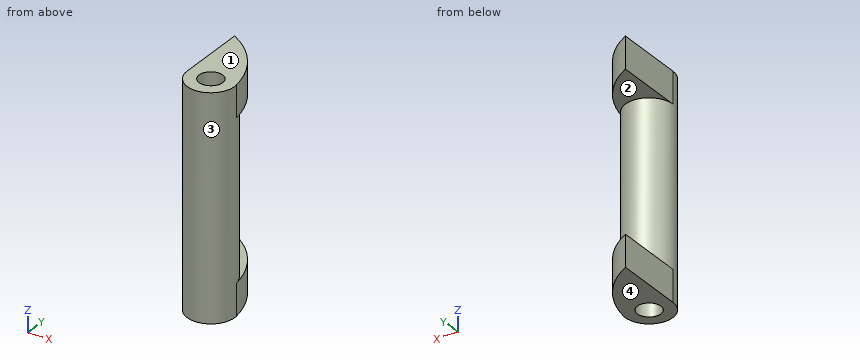
Autodesk Inventor part; units mm, degrees
ref_plane "YZ Plane" through (0, 0, 0) normal (1, 0, 0) x (0, 1, 0)
ref_plane "XZ Plane" through (0, 0, 0) normal (0, 1, 0) x (-1, 0, 0)
sketch "草图1" plane through (0, 0, 0) normal (0, 0, 1) x (1, 0, 0)
  circle A0 centre (0, 0) radius 1.5
  circle A1 centre (0, 0) radius 3
  line L0 (-3, 0) -> (-3, 9)
  arc A2 (2.9736, 0.3973) -> (-3, 9) centre (-8.3955, -1.1218) ccw
  dimension "d0" = 3
  dimension "d1" = 6
  dimension "d2" = 9
sketch "草图2" plane through (0, 0, 0) normal (0, 1, 0) x (-1, 0, 0)
  line L0 (3, 0) -> (3, -28)
  line L1 (3, 0) -> (3, -4)
  line L2 (3, -28) -> (3, -24)
  point P0 (0, 0)
  point P1 (3, -14)
  dimension "d3" = 28
  dimension "d6" = 4
  dimension "d7" = 4
extrude "拉伸1" add sketch "草图1" against normal blind 28 contours A1
extrude "拉伸2" add sketch "草图1" against normal blind 4 contours A1 L0 A2
ref_plane "工作平面1" through (0, 0, -14) normal (0, 0, 1) x (1, 0, 0)
mirror "镜像1" about plane through (0, 0, -14) normal (0, 0, 1) of "拉伸2"
thread "螺纹8"
Model file for the job. Use its own axes, mm. Face numbers are marked on the shaded views. Round coordinates to 2 decimals unless told otherwise and drop trailing zeros. Order: outer loops, then holes, each group sorted by start corner. A loop starts at its lowest first (then second) coordinate and runs counter-clockwise, first axis right, second up.
(1) Drill centre lines: line 1 (Y direction, x = 0, z = -7.5); line 2 (Z direction, x = -1.65, y = 3.25); line 3 (Y direction, x = 0, z = -25.25). Where is each one in solid material? Low to high.
(2) Band-saw the part on B-B (x = 0). List the corners of the cut face in (y, z).
(3) Band-saw the part on D-D (y = -1). List the corners of the cut face in (x, z).
(4) Band-saw the part on A-A (y = 1). List the corners of the cut face in (x, z).
(5) Pull direction Z, two halves, no side cores. Call the marked faces 1, 2, 3 and 4: released by +Z, released by -Z, zero draft, split by the parting line, or undercut.
(6) Band-saw the part on C-C (z = -1.5). List the corners of the cut face in (x, y), then the cut area to 3 significant figures.
Verdict:
1. line 1: y = -3 to -1.5, 1.5 to 3
1. line 2: z = -28 to -24, -4 to 0
1. line 3: y = -3 to -1.5, 1.5 to 6.69
2. outline: (-3, -28) - (-1.5, -28) - (-1.5, 0) - (-3, 0) - close; (1.5, -28) - (6.69, -28) - (6.69, -24) - (3, -24) - (3, -4) - (6.69, -4) - (6.69, 0) - (1.5, 0) - close
3. outline: (-2.83, -28) - (-1.12, -28) - (-1.12, 0) - (-2.83, 0) - close; (1.12, -28) - (2.83, -28) - (2.83, 0) - (1.12, 0) - close
4. outline: (-3, -28) - (-1.12, -28) - (-1.12, 0) - (-3, 0) - (-3, -4) - (-2.83, -4) - (-2.83, -24) - (-3, -24) - close; (1.12, -28) - (2.88, -28) - (2.88, -24) - (2.83, -24) - (2.83, -4) - (2.88, -4) - (2.88, 0) - (1.12, 0) - close
5. face 1: released by +Z
5. face 2: undercut
5. face 3: undercut
5. face 4: released by -Z
6. outline: (-3, 0) arc R3 ccw (long way) to (2.97, 0.4) arc R11.47 ccw to (-3, 9) - close; hole circle Ø3 at (0, 0)
6. area: 44.1 mm2
